```python
from build123d import *

# Parameters (mm, degrees)
HOLE_WIZARD_M3_1_D = 2.5
CHAMFER_1_SIZE     = 0.5


with BuildPart() as part:
    # 草图1 → 旋转1 (revolve)
    with BuildSketch(Plane.XY, mode=Mode.PRIVATE) as revolve_1_sk:
        Polygon((0, 0), (0, 40), (2.5, 40), (2.5, 28), (3.5, 28), (3.5, 23), (4, 23), (4, 21), (10, 21), (10, 11), (4, 11), (4, 9), (3.5, 9), (3.5, 4), (2.5, 4), (2.5, 0), align=None)
    revolve(revolve_1_sk.sketch.rotate(Axis((0, 0, 0), (0, 1, 0)), 90), axis=Axis((0, 0, 0), (0, 1, 0)))

    # M3 螺纹孔1 (through all)
    with Locations(Plane(origin=(0, 21, 0), x_dir=(1, 0, 0), z_dir=(0, 1, 0))):
        with Locations((0, 7), (7, 0), (0, -7), (-7, 0)):
            Hole(HOLE_WIZARD_M3_1_D / 2)

    # 倒角1
    chamfer_1_edges = [part.edges().sort_by_distance(p)[0] for p in [
        (0, 0, 2.5),
        (0, 40, 2.5),
    ]]
    chamfer(chamfer_1_edges, length=CHAMFER_1_SIZE)


solid = part.part
```
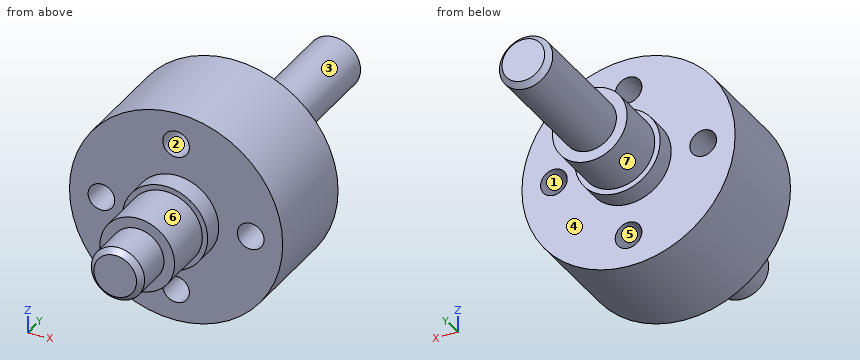
Geometry: final body of the model. Coordinates: model frame, mm. Face numbers are marked on the shaded views. A direction names the side the tool comes from. Give positions to 0.01 mm unless a question says otherwise; leave off trailing zeros. Order: outer loops, then holes, each group sorted by start corner. A loop starts at its lowest first (then second) coordinate and runs counter-clockwise, first axis right, second up. Notation, with made-up numbers: (6.5, 8.5) -> (43.5, 8.5) arc R7 ccw to (43.5, 14.5) -> close; hole circle Ø6 at (40.25, 38.5). An arc over 180 degrees is marked (long way). Write each question's results on one line, items separated by ' | '. Start each with the question number.
1) Section C-C (z = 7). Return loops of the section in (x, y).
2) Set-up query: the marked faces 5, 6 and 7. Return all of +Z, -Z, +X, -X, +Y, -Y with unobstructed straight access to the full face (end or side cutting, diameter ignored); none if empty.
3) First-contact query: pin 1 (6 mm diameter, centred on y = 15.5, z = 5, fed in from +X); pin 2 (1.5 mm diameter, centred on x = 5.5, z = 6, fed in from +Y); pin 3 (1 mm diameter, centred on x = -2.5, y = 22, fed in from +Z); pin 4 (2 mm diameter, centred on x = 7, z = 0, fed in from +Y). Flat tips, straight axial feed; report the tip coordinate or a pass-through.
4) Draft query along X for the marked faces 1, 2, 3 and 4. Return one class per face: pulls with the +X half, pulls with the -X half, needs draft (parallel to the pull), parting line crosses it, or undercut.
5) Section B-B (y = 15.5). Return loops of the section in (x, z), then the cut area to 3 significant figures.
6) Section A-A (x = -7). Return loops of the section in (y, z).
7) Section D-D (x = 0). Count the separate pieces of the cut face and the enclosed holes in it, then the cut area to 4 significant figures.
8) Line query: line 1 (Y direction, x = 1.75, z = -6.25); line 2 (X direction, y = 16.5, z = 6.25); line 3 (X direction, y = 28.5, z = -1.25). Output: solid intervals per line, ascending. Write a range as from..to.
Calculated:
1) outline: (-7.14, 11) -> (-1.25, 11) -> (-1.25, 21) -> (-7.14, 21) -> close; (1.25, 11) -> (7.14, 11) -> (7.14, 21) -> (1.25, 21) -> close
2) face 5: +Y, -Y | face 6: -Y | face 7: +Y
3) pin 1: x = 9.8 | pin 2: y = 21 | pin 3: z = 3.46 | pin 4: through
4) face 1: undercut | face 2: undercut | face 3: parting line crosses it | face 4: needs draft
5) outline: circle Ø20 at (0, 0); hole circle Ø2.5 at (-7, 0); hole circle Ø2.5 at (0, -7); hole circle Ø2.5 at (0, 7); hole circle Ø2.5 at (7, 0) | area: 295 mm2
6) outline: (11, -7.14) -> (21, -7.14) -> (21, -1.25) -> (11, -1.25) -> close; (11, 1.25) -> (21, 1.25) -> (21, 7.14) -> (11, 7.14) -> close
7) separate pieces: 3 | enclosed holes: 0 | area: 331.5 mm2
8) line 1: 11..21 | line 2: -7.81..-1, 1..7.81 | line 3: -2.17..2.17
